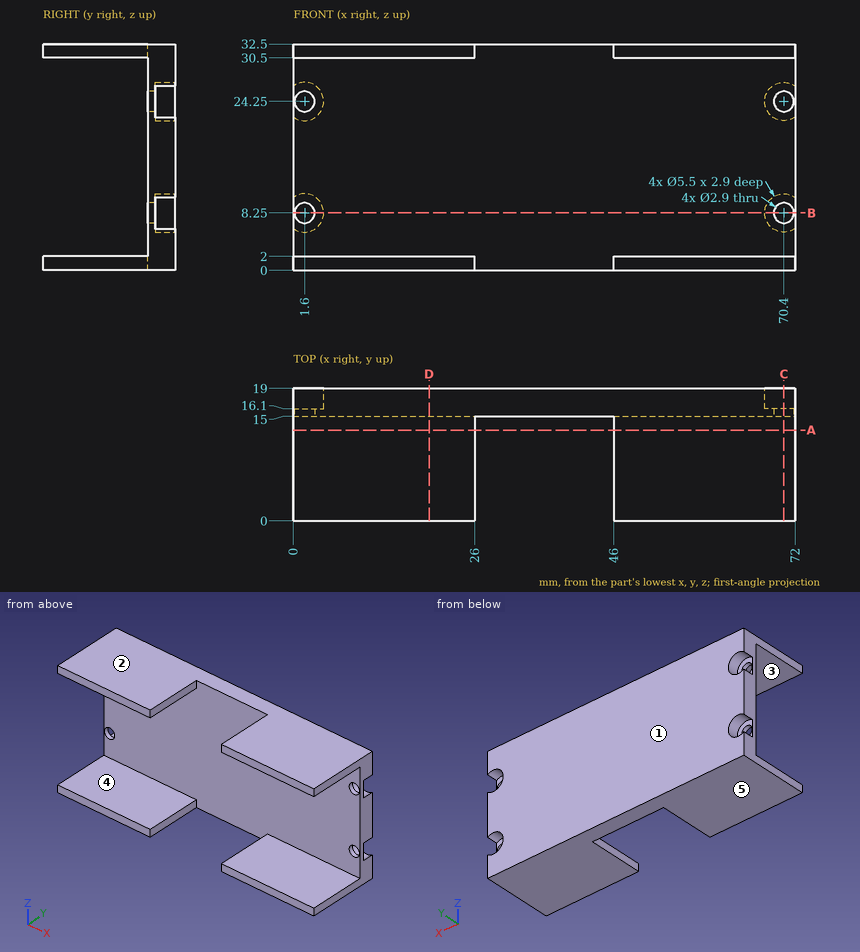
Can you work these out from the drawing? Everything is in mm from the part's minimum corner. A direction names the side the tool comes from. Round coordinates to 2 decimals unless told otherwise and drop trailing zeros. Order: outer loops, then holes, each group sorted by start corner. A loop starts at its lowest first (then second) coordinate and runs counter-clockwise, first axis right, second up. Notation, with made-up numbers: M 31.5,-17 L 79.5,-17 A29 cw 79.5,11 Z; hole C 22.25,38.25 d3. An arc over 180 degrees is marked long. Answer as CSV lines item,"result".
Item 1: For pin 1 (4 mm diameter, centred on x = 1.6, z = 8.25, fed in from -Y); pin 2 (2 mm diameter, centred on x = 2, z = 25, fed in from +Y), each with a flat end and sliding along its axis, tell me the tip position at first contact or that it passes through.
From the geometry:
pin 1,"y = 15"
pin 2,"y = 16.1"
Item 2: Imagine slicing it at A-A on y = 13. List the corners of the cut face in (x, z) for me.
From the geometry:
outline,"M 0,0 L 26,0 L 26,2 L 0,2 Z; M 0,30.5 L 26,30.5 L 26,32.5 L 0,32.5 Z; M 46,0 L 72,0 L 72,2 L 46,2 Z; M 46,30.5 L 72,30.5 L 72,32.5 L 46,32.5 Z"
Item 3: Imagine slicing it at B-B on z = 8.25. List the corners of the cut face in (x, y) for me.
From the geometry:
outline,"M 0,15 L 0.15,15 L 0.15,16.1 L 0,16.1 Z; M 3.05,15 L 68.95,15 L 68.95,16.1 L 67.65,16.1 L 67.65,19 L 4.35,19 L 4.35,16.1 L 3.05,16.1 Z; M 71.85,15 L 72,15 L 72,16.1 L 71.85,16.1 Z"
Item 4: Imagine slicing it at D-D on x = 19.5. List the corners of the cut face in (y, z) for me, and give its area (3 significant figures).
From the geometry:
outline,"M 0,0 L 19,0 L 19,32.5 L 0,32.5 L 0,30.5 L 15,30.5 L 15,2 L 0,2 Z"
area,"190 mm2"
Item 5: Please list where these lines run through material, in increasing order: L1, parallel to Z at x = 70.4, y = 17.4; L2, parallel to Z at x = 1.6, y = 15.7; L3, parallel to X at y = 15.8, z = 8.25. Write a range as [from, to].
From the geometry:
L1,"[0, 5.5], [11, 21.5], [27, 32.5]"
L2,"[0, 6.8], [9.7, 22.8], [25.7, 32.5]"
L3,"[0, 0.15], [3.05, 68.95], [71.85, 72]"
Item 6: Imagine slicing it at C-C on x = 70.4. List the corners of the cut face in (y, z) for me.
From the geometry:
outline,"M 0,0 L 19,0 L 19,5.5 L 16.1,5.5 L 16.1,6.8 L 15,6.8 L 15,2 L 0,2 Z; M 0,30.5 L 15,30.5 L 15,25.7 L 16.1,25.7 L 16.1,27 L 19,27 L 19,32.5 L 0,32.5 Z; M 15,9.7 L 16.1,9.7 L 16.1,11 L 19,11 L 19,21.5 L 16.1,21.5 L 16.1,22.8 L 15,22.8 Z"
Item 7: Which directions (+Z, -Z, +X, -X, +Y, -Y) give clear straight access to the entire face, cutting with the end or side of a thin tool? Please do the marked faces 4 and 5.
From the geometry:
face 4,"+X, -X, -Y"
face 5,"-Z, +X, -X, +Y, -Y"
Item 8: We'd pull the mould along Z, two halves only. Please class the marked faces 1, 2 and 3: +Z half, -Z half, draft (parallel to the pull), parting line (faces both ways), or undercut.
From the geometry:
face 1,"draft"
face 2,"+Z half"
face 3,"undercut"
